Verification items for the finished model (mm, model axes). A direction names the side the tool comes from. Coordinates: 2 decimals unless noted, no trailing zeros. Order: outer loops, then holes, each group sorted by start corner. A loop starts at its lowest first (then second) coordinate and runs counter-clockwise, first axis right, second up. Notation, with made-up numbers: M -19.5,67 L 7.5,67 A36 cw 7.5,102 Z; hole C 58.5,51 d7. An arc over 180 degrees is marked long. Return JSON: item names as keys, results as strings.
```python
from build123d import *

# Parameters (mm, degrees)
SKETCH1_R          = 88.773
BASE_DEPTH         = 6.35
STOPPER_DEPTH      = 12.7
STOPPER_START      = -6.35
STOPPER_GAP_DEPTH  = 13.7
OVERHANG_CUT_DEPTH = 26.416
CIRPATTERN1_COUNT  = 4


with BuildPart() as part:
    # Sketch1 → Base (new body)
    with BuildSketch(Plane(origin=(0, 0, 0), x_dir=(1, 0, 0), z_dir=(0, 1, 0))):
        Circle(SKETCH1_R)
    extrude(amount=BASE_DEPTH)

    # Sketch2 → Stopper (add)
    with BuildSketch(Plane(origin=(0, 6.35, 0), x_dir=(1, 0, 0), z_dir=(0, 1, 0))):
        with BuildLine():
            Line((-44.45, -76.842976445), (-44.45, -51.442976445))
            Line((-44.45, -51.442976445), (0, -51.442976445))
            Line((0, -51.442976445), (44.45, -51.442976445))
            Line((44.45, -51.442976445), (44.45, -76.842976445))
            ThreePointArc((44.45, -76.842976445), (23.011562105, -85.73863504), (0, -88.773))
            ThreePointArc((0, -88.773), (-23.011562105, -85.73863504), (-44.45, -76.842976445))
        make_face()
    stopper = extrude(amount=STOPPER_DEPTH)

    # Sketch5 → Stopper Gap (cut, through all)
    with BuildSketch(Plane(origin=(0, 19.05, 0), x_dir=(1, 0, 0), z_dir=(0, 1, 0)).offset(STOPPER_START)):
        with BuildLine():
            Line((-38.10000012, -80.181266639), (-38.10000012, -51.442976445))
            Line((-38.10000012, -51.442976445), (-1.2e-07, -51.442976445))
            Line((-1.2e-07, -51.442976445), (38.09999988, -51.442976445))
            Line((38.09999988, -51.442976445), (38.10000012, -80.181266639))
            ThreePointArc((38.10000012, -80.181266639), (19.528363291, -86.598432758), (0, -88.773))
            ThreePointArc((0, -88.773), (-19.528363291, -86.598432758), (-38.10000012, -80.181266639))
        make_face()
    stopper_gap = extrude(amount=-STOPPER_GAP_DEPTH, mode=Mode.SUBTRACT)

    # Sketch6 → Overhang cut (cut)
    with BuildSketch(Plane(origin=(0, 19.05, 0), x_dir=(1, 0, 0), z_dir=(0, 1, 0))):
        with BuildLine():
            Line((-25.4, -51.442976445), (0, -51.442976445))
            Line((0, -51.442976445), (25.4, -51.442976445))
            Line((25.4, -51.442976445), (44.45, -51.442976445))
            Line((44.45, -51.442976445), (44.45, -56.522976445))
            Line((44.45, -56.522976445), (25.4, -56.522976445))
            Line((25.4, -56.522976445), (25.4, -85.06165722))
            ThreePointArc((25.4, -85.06165722), (12.834855523, -87.840264188), (0, -88.773))
            ThreePointArc((0, -88.773), (-12.834855523, -87.840264188), (-25.4, -85.06165722))
            Line((-25.4, -85.06165722), (-25.4, -56.522976445))
            Line((-25.4, -56.522976445), (-44.45, -56.522976445))
            Line((-44.45, -56.522976445), (-44.45, -51.442976445))
            Line((-44.45, -51.442976445), (-25.4, -51.442976445))
        make_face()
    overhang_cut = extrude(amount=-OVERHANG_CUT_DEPTH, mode=Mode.SUBTRACT)

    # CirPattern1: Stopper, Stopper Gap, Overhang cut ×4 about axis
    cirpattern1_axis = Axis((0, 0, 0), (0, 1, 0))
    for i in range(1, CIRPATTERN1_COUNT):
        add(stopper.rotate(cirpattern1_axis, i * 360 / CIRPATTERN1_COUNT))
        add(stopper_gap.rotate(cirpattern1_axis, i * 360 / CIRPATTERN1_COUNT), mode=Mode.SUBTRACT)
        add(overhang_cut.rotate(cirpattern1_axis, i * 360 / CIRPATTERN1_COUNT), mode=Mode.SUBTRACT)


solid = part.part
```
Q1. Go/stop test with flat-tipped pins: pin 1 (6.5 mm diameter, centred on y = 9, z = 64.5, fed in from +X); pin 2 (5 mm diameter, centred on x = 67, y = 17, fed in from +Z); pin 3 (4 mm diameter, centred on y = 9, z = -65.5, fed in from +X). Record where each tip stops, or that it passes through.
Values:
{"pin 1": "x = 62.93", "pin 2": "z = 44.45", "pin 3": "x = 44.45"}
Q2. Cross-section at A-A, the plane y = 9.5. State how many separate pieces and enclosed holes the cut face has, and give its area (3 significant figures).
Values:
{"separate pieces": "8", "enclosed holes": "0", "area": "1,120 mm^2"}
Q3. Draft check along X on faces 1 (the face through (-38.1, 6, 69)), 2 (the face through (35, 19.05, -71)), 3 (the face through (-44.45, 13, 67)). Enter one of: pulls with the +X half, pulls with the -X half, needs draft (parallel to the pull), parting line crosses it, or undercut.
Values:
{"face 1": "undercut", "face 2": "needs draft", "face 3": "pulls with the -X half"}
Q4. Cross-section at D-D, the plane z = 12. Record the boundary of the cut face in (x, y), and give its area (3 significant figures).
Values:
{"outline": "M -51.44,0 L 51.44,0 L 51.44,6.35 L -51.44,6.35 Z", "area": "653 mm^2"}
Q5. Material ranges on line 1 along X through (y, z) = (18.25, -69); line 2 along Z through (x, y) = (68, 6.75), recorded low to high.
Values:
{"line 1": "-44.45 to -25.4, 25.4 to 44.45", "line 2": "-44.45 to -38.1, 38.1 to 44.45"}
Q6. Tool access check on faces 4 (the face through (-37, 14, -56.523)), 5 (the face through (25.4, 16, 71)), 6 (the face through (69, 6, 38.1)), 7 (the face through (-32, 12.7, 71)). Record the directions out of +Z, -Z, +X, -X, +Y, -Y that give a thin tool (end or side, any length) a straight path to the whole face; none if there is none.
Values:
{"face 4": "+Y, -Y", "face 5": "+Z, -Z, +Y, -Y", "face 6": "+X, -Y", "face 7": "+Z, -Z, -Y"}
Q7. Cross-section at B-B, the plane x = 64. Record the boundary of the cut face in (y, z).
Values:
{"outline": "M 0,-61.52 L 6.35,-61.52 L 6.35,-44.45 L 19.05,-44.45 L 19.05,-25.4 L 12.7,-25.4 L 12.7,-38.1 L 0,-38.1 Z; M 0,38.1 L 12.7,38.1 L 12.7,25.4 L 19.05,25.4 L 19.05,44.45 L 6.35,44.45 L 6.35,61.52 L 0,61.52 Z"}
Q8. Cross-section at C-C, the plane x = 5. Record the boundary of the cut face in (y, z).
Values:
{"outline": "M 0,-51.44 L 6.35,-51.44 L 6.35,51.44 L 0,51.44 Z"}
